from build123d import *

# Parameters (mm, degrees)
F0_R     = 20
F0_R_2   = 4.999997
F1_DEPTH = 25
F2_SIZE  = 2


with BuildPart() as f1:
    # F0 (on Front) → F1 (new body)
    with BuildSketch(Plane.XZ):
        with BuildLine():
            ThreePointArc((10.867925, -27.962264), (24.759218, -16.940517), (30, 0))
            ThreePointArc((30, 0), (21.213203, 21.213203), (0, 30))
            ThreePointArc((0, 30), (-29.486166, -5.528656), (10.867925, -27.962264))
        make_face()
        Circle(F0_R, mode=Mode.SUBTRACT)
        with BuildLine():
            ThreePointArc((0, 30), (21.213203, 21.213203), (30, 0))
            ThreePointArc((30, 0), (24.759218, -16.940517), (10.867925, -27.962264))
            Line((10.867925, -27.962264), (85.433962, 1.018868))
            ThreePointArc((85.433962, 1.018868), (65.256917, 12.235672), (80, 30))
            Line((80, 30), (0, 30))
        make_face()
        with BuildLine():
            ThreePointArc((95, 15), (90.606602, 25.606602), (80, 30))
            ThreePointArc((80, 30), (65.256917, 12.235672), (85.433962, 1.018868))
            ThreePointArc((85.433962, 1.018868), (92.379609, 6.529741), (95, 15))
        make_face()
        with Locations((80, 15)):
            Circle(F0_R_2, mode=Mode.SUBTRACT)
    extrude(amount=F1_DEPTH)

    # F2
    f2_edges = [f1.edges().sort_by_distance(p)[0] for p in [
        (-20, -25, 0),
        (75.000003, -25, 15),
        (-20, 0, 0),
        (75.000003, 0, 15),
        (40, 0, 30),
        (40, -25, 30),
    ]]
    chamfer(f2_edges, length=F2_SIZE)


solid = f1.part
Check sheet for the modelled part. Datum: model origin and axes. Units: mm. Coordinates: 2 decimals unless noted, no trailing zeros. Loops run counter-clockwise (first coordinate to the right, second up) from the corner with the lowest first, then second, coordinate; pieces in that order, holes last. Notation, with made-up numbers: (46, 45) -> (78, 45) arc R24 cw to (78, 64) -> close; hole circle Ø6 at (10.5, 55). An arc over 180 degrees is marked (long way). Write item = value, one per line. Start each with the question number.
1. Section check C-C on x = 46. Record the cut outline in (y, z), then the cut area to 3 significant figures.
2. Section check B-B on x = 66. Record the cut outline in (y, z), then the cut area to 3 significant figures.
3. Section check A-A on y = -4. Record the cut outline in (x, z).
4. Material ranges on line 1 (Z direction, x = 0, y = -9.75); line 2 (X direction, y = -20.5, z = 18); line 3 (X direction, y = -12, z = 12), recorded low to high.
5. Depth check by flat-ended pin: P1, Ø9, axis at x = 80, z = 15, coming from the +Y side; P2, Ø2, axis at y = -6, z = -12, coming from the -X side; P3, Ø1.5, axis at x = 75, y = -6, coming from the -Z side; P4, Ø8, axis at y = -20.5, z = 19.5, coming from the +X side. Enter the tip coordinate at first touch or a pass-through.
6. Draft check along Z on faces 1 (the flat face through (32, -25, 7)), 2 (the flat face through (47.262, -24.014, -12.729)), 3 (the conical face through (84.888, -23.125, 16.539)). Enter one of: released by +Z, released by -Z, zero draft, split by the parting line, or undercut.
Responses:
q1.outline = (-25, -12.16) -> (-23, -14.31) -> (-2, -14.31) -> (0, -12.16) -> (0, 28) -> (-2, 30) -> (-23, 30) -> (-25, 28) -> close
q1.area = 1,100 mm2
q2.outline = (-25, -4.39) -> (-23, -6.53) -> (-2, -6.53) -> (0, -4.39) -> (0, 28) -> (-2, 30) -> (-23, 30) -> (-25, 28) -> close
q2.area = 905 mm2
q3.outline = (0, 30) arc R30 ccw (long way) to (10.87, -27.96) -> (85.43, 1.02) arc R15 ccw to (95, 15) arc R15 ccw to (80, 30) -> close; hole circle Ø40 at (0, 0); hole circle Ø10 at (80, 15)
q4.line_1 = -30 to -20, 20 to 30
q4.line_2 = -24 to -8.72, 8.72 to 76, 84 to 94.7
q4.line_3 = -27.5 to -16, 16 to 76, 84 to 94.7
q5.P1 = through
q5.P2 = -27.91
q5.P3 = -3.33
q5.P4 = 94.99
q6.face_1 = zero draft
q6.face_2 = released by -Z
q6.face_3 = undercut
